Read the model definition and answer for the solid it produces. Units are mm, in the model's axes. Coordinates: 2 decimals unless noted, no trailing zeros. Write each loop counter-clockwise with the first axis right and the second up, starting at its lowest first coordinate (ties: lowest second). Pieces come first, ordered by that corner, then holes. Notation, with made-up numbers: (-9, 18) -> (34, 18) arc R13 cw to (34, 31) -> close; hole circle Ø3 at (53.25, 38.25). An arc over 180 degrees is marked (long way). Answer in a Markdown table with one row per item. Add a question column.
Item 1: Section B-B on z = -323 is taken. Write down the section's boundary in (x, y).
Item 2: Section C-C on x = 332.5 is taken. Write down the section's boundary in (y, z).
Item 3: Given pin 1 Ø1.5 at (x, y) = (257, 1.5) entering from -Z, flat-ended and moving along its own axis, determine where the tip first touches the part or whether it passes through.
Item 4: Section A-A on y = 2.2 is taken. Write down the section's boundary in (x, z), then the cut area to 3 significant figures.
Item 5: Straight lines are drawn through the part: line 1 (X direction, y = 1.3, z = -10); line 2 (Z direction, x = 160, y = 0.65); line 3 (X direction, y = 2.3, z = -304). For each, find the intervals that lie inside material, in ascending order. Write a range as from..to.
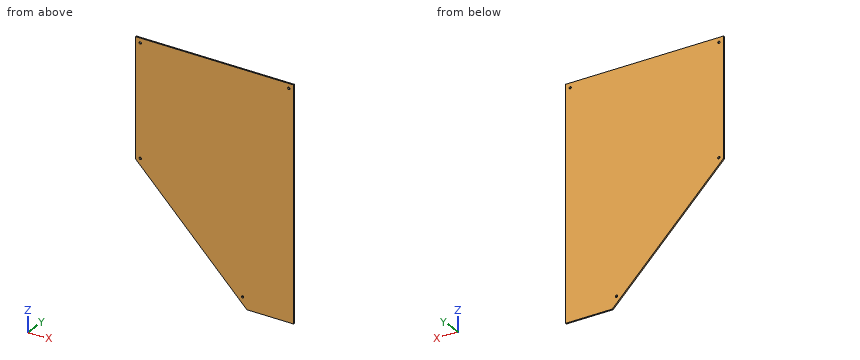
```python
from build123d import *

# Parameters (mm, degrees)
BOSS_EXTRUDE1_DEPTH  = 3
SKETCH3_R            = 2.5
MOUNTING_HOLES_DEPTH = 4


with BuildPart() as part:
    # Sketch2 → Boss-Extrude1 (new body)
    with BuildSketch(Plane(origin=(0, 0, 0), x_dir=(1, 0, 0), z_dir=(0, 1, 0))):
        Polygon((150, 250), (388.61, 488.61), (488.61, 488.61), (488.61, 0), (150, 0), align=None)
    extrude(amount=BOSS_EXTRUDE1_DEPTH)

    # Sketch3 → mounting-holes (cut, through all)
    with BuildSketch(Plane(origin=(0, 3, 0), x_dir=(1, 0, 0), z_dir=(0, 1, 0))):
        with Locations((160, 245.857864376)):
            Circle(SKETCH3_R)
        with Locations((160, 10)):
            Circle(SKETCH3_R)
        with Locations((478.61, 10)):
            Circle(SKETCH3_R)
        with Locations((379.368855681, 465.226720057)):
            Circle(SKETCH3_R)
    extrude(amount=-MOUNTING_HOLES_DEPTH, mode=Mode.SUBTRACT)


solid = part.part
```
Results below:
| question | item | result |
|---|---|---|
| 1 | outline | (223, 0) -> (488.61, 0) -> (488.61, 3) -> (223, 3) -> close |
| 2 | outline | (0, -432.5) -> (3, -432.5) -> (3, 0) -> (0, 0) -> close |
| 3 | pin 1 | stops at z = -357.75 |
| 4 | outline | (150, -250) -> (388.61, -488.61) -> (488.61, -488.61) -> (488.61, 0) -> (150, 0) -> close; hole circle Ø5 at (160, -245.86); hole circle Ø5 at (160, -10); hole circle Ø5 at (379.37, -465.23); hole circle Ø5 at (478.61, -10) |
| 4 | area | 137,000 mm2 |
| 5 | line 1 | x = 150..157.5, 162.5..476.11, 481.11..488.61 |
| 5 | line 2 | z = -260..-248.36, -243.36..-12.5, -7.5..0 |
| 5 | line 3 | x = 204..488.61 |
